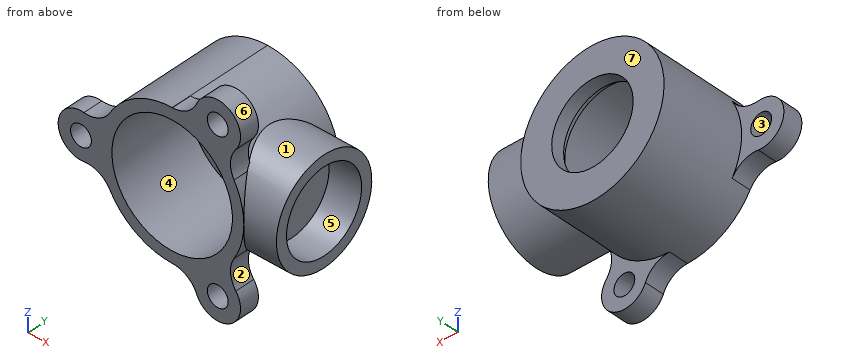
from build123d import *
from build123d.topology import SkipClean

# Parameters (mm, degrees)
SKETCH_1_R          = 11
EXTRUDE_1_DEPTH     = 16
CUT_EXTRUDE_1_REACH = 24.316
SKETCH_2_R          = 6.25
SKETCH_3_R          = 9.25
CUT_EXTRUDE_2_DEPTH = 13
EXTRUDE_2_REACH     = 35.257
SKETCH_4_R          = 8
SKETCH_5_R          = 6.3
CUT_EXTRUDE_3_DEPTH = 5
SKETCH_6_R          = 1.6
EXTRUDE_3_DEPTH     = 3
SKETCH_7_R          = 7
CUT_EXTRUDE_4_DEPTH = 1


with BuildPart() as part:
    # 草图1 → 凸台-拉伸1 (new body)
    with BuildSketch(Plane(origin=(0, 0, 0), x_dir=(1, 0, 0), z_dir=(0, 1, 0))):
        with Locations(Location((0, 0, 0), (0, 0, 270))):
            Circle(SKETCH_1_R)
    extrude(amount=EXTRUDE_1_DEPTH)

    # 草图2 → 切除-拉伸1 (cut, up to next)
    with BuildSketch(Plane(origin=(0, 16, 0), x_dir=(1, 0, 0), z_dir=(0, 1, 0)), mode=Mode.PRIVATE) as cut_extrude_1_sk1:
        with Locations(Location((0, 0, 0), (0, 0, 270))):
            Circle(SKETCH_2_R)
    cut_extrude_1_tool1 = extrude(cut_extrude_1_sk1.sketch, amount=-CUT_EXTRUDE_1_REACH, mode=Mode.PRIVATE) & part.part
    add(cut_extrude_1_tool1.solids().sort_by_distance((0, 16, 0))[0], mode=Mode.SUBTRACT)

    # 草图3 → 切除-拉伸2 (cut)
    with BuildSketch(Plane.XZ):
        with Locations(Location((0, 0, 0), (0, 0, 270))):
            Circle(SKETCH_3_R)
    extrude(amount=-CUT_EXTRUDE_2_DEPTH, mode=Mode.SUBTRACT)

    # 草图4 → 凸台-拉伸2 (add, up to next)
    with BuildSketch(Plane(origin=(16, 0, 0), x_dir=(0, 0, -1), z_dir=(1, 0, 0)), mode=Mode.PRIVATE) as extrude_2_sk1:
        with Locations((0, 8)):
            Circle(SKETCH_4_R)
    extrude_2_tool1 = extrude(extrude_2_sk1.sketch, amount=-EXTRUDE_2_REACH, mode=Mode.PRIVATE) - part.part
    add(extrude_2_tool1.solids().sort_by_distance((16, 8, 0))[0])

    # 草图5 → 切除-拉伸3 (cut)
    with SkipClean():  # the faces are left unmerged after this step: merging them gives an invalid solid
        with BuildSketch(Plane(origin=(16, 0, 0), x_dir=(0, 0, -1), z_dir=(1, 0, 0))):
            with Locations((0, 8)):
                Circle(SKETCH_5_R)
        extrude(amount=-CUT_EXTRUDE_3_DEPTH, mode=Mode.SUBTRACT)

    # 草图6 → 凸台-拉伸3 (add)
    # profile 1 of 3: a face of its own
    with SkipClean():  # the faces are left unmerged after this step: merging them gives an invalid solid
        with BuildSketch(Plane.XZ):
            with BuildLine():
                ThreePointArc((-11, 0), (-10.632091471, 2.821104562), (-9.55297619, 5.453498501))
                ThreePointArc((-9.55297619, 5.453498501), (-11.247511613, 3.854105973), (-13.545833333, 3.470408137))
                ThreePointArc((-13.545833333, 3.470408137), (-17.5, 0), (-13.545833333, -3.470408137))
                ThreePointArc((-13.545833333, -3.470408137), (-11.247511613, -3.854105973), (-9.55297619, -5.453498501))
                ThreePointArc((-9.55297619, -5.453498501), (-10.632091471, -2.821104562), (-11, 0))
            make_face()
            with Locations(Location((-14, 0, 0), (0, 0, 270))):
                Circle(SKETCH_6_R, mode=Mode.SUBTRACT)
        # profile 2 of 3: a face of its own
        with BuildSketch(Plane.XZ):
            with BuildLine():
                ThreePointArc((9.778378275, 9.995831713), (8.75, 15.155444566), (3.767455058, 13.466239851))
                ThreePointArc((3.767455058, 13.466239851), (2.286002125, 11.667683773), (0.053619854, 10.999869313))
                ThreePointArc((0.053619854, 10.999869313), (5.5, 9.526279442), (9.499356337, 5.546370812))
                ThreePointArc((9.499356337, 5.546370812), (8.961509488, 7.8135778), (9.778378275, 9.995831713))
            make_face()
            with Locations(Location((7, 12.124355653, 0), (0, 0, 270))):
                Circle(SKETCH_6_R, mode=Mode.SUBTRACT)
        # profile 3 of 3: a face of its own
        with BuildSketch(Plane.XZ):
            with BuildLine():
                ThreePointArc((3.767455058, -13.466239851), (8.75, -15.155444566), (9.778378275, -9.995831713))
                ThreePointArc((9.778378275, -9.995831713), (8.961509488, -7.8135778), (9.499356337, -5.546370812))
                ThreePointArc((9.499356337, -5.546370812), (5.5, -9.526279442), (0.053619854, -10.999869313))
                ThreePointArc((0.053619854, -10.999869313), (2.286002125, -11.667683773), (3.767455058, -13.466239851))
            make_face()
            with Locations(Location((7, -12.124355653, 0), (0, 0, 270))):
                Circle(SKETCH_6_R, mode=Mode.SUBTRACT)
        extrude(amount=-EXTRUDE_3_DEPTH)

    # 草图7 → 切除-拉伸4 (cut)
    with SkipClean():  # the faces are left unmerged after this step: merging them gives an invalid solid
        with BuildSketch(Plane.XZ.offset(-13)):
            with Locations(Location((0, 0, 0), (0, 0, 270))):
                Circle(SKETCH_7_R)
        extrude(amount=-CUT_EXTRUDE_4_DEPTH, mode=Mode.SUBTRACT)


solid = part.part
The listing builds one solid part. Answer for the finished solid, in the listing's coordinates (mm). Face numbers are marked on the shaded views. A direction names the side the tool comes from. Round coordinates to 2 decimals unless told otherwise and drop trailing zeros. Order: outer loops, then holes, each group sorted by start corner. A loop starts at its lowest first (then second) coordinate and runs counter-clockwise, first axis right, second up. Notation, with made-up numbers: (12.5, 72) -> (53.5, 72) arc R21 ccw to (53.5, 84) -> close; hole circle Ø3 at (33.5, -3). An arc over 180 degrees is marked (long way). One line per item, written item: value.
Item 1: Straight lines are drawn through the part: L1, parallel to X at y = 2, z = -0.5; L2, parallel to Z at x = 9.5, y = 14; L3, parallel to X at y = 14.5, z = 0. For each, find the intervals that lie inside material, in ascending order.
Taken from the geometry:
L1: x = -17.46 to -15.52, -12.48 to -9.24, 9.24 to 11
L2: z = -5.55 to 5.55
L3: x = -11 to -6.25, 6.25 to 16
Item 2: Find section A-A, the plane x = -14. Give the vertices of the cut face in (y, z), then the cut area to 3 significant figures.
Taken from the geometry:
outline: (0, -3.5) -> (3, -3.5) -> (3, -1.6) -> (0, -1.6) -> close; (0, 1.6) -> (3, 1.6) -> (3, 3.5) -> (0, 3.5) -> close
area: 11.4 mm2
Item 3: Find section C-C, the plane z = -5. Give the vertices of the cut face in (x, y) (3 decimals), then the cut area to 3 significant figures.
Taken from the geometry:
outline: (-9.855, 0) -> (-7.782, 0) -> (-7.782, 13) -> (-4.899, 13) -> (-4.899, 14) -> (-3.75, 14) -> (-3.75, 16) -> (-9.798, 16) -> (-9.798, 3) -> (-9.855, 3) -> close; (3.75, 14) -> (4.899, 14) -> (4.899, 13) -> (7.782, 13) -> (7.782, 0) -> (9.798, 0) -> (9.798, 1.755) -> (16, 1.755) -> (16, 4.167) -> (11, 4.167) -> (11, 11.833) -> (16, 11.833) -> (16, 14.245) -> (9.798, 14.245) -> (9.798, 16) -> (3.75, 16) -> close
area: 126 mm2
Item 4: Find section D-D, the plane z = 8.5. Give the vertices of the cut face in (x, y), then the cut area to 3 significant figures.
Taken from the geometry:
outline: (-6.98, 0) -> (-3.65, 0) -> (-3.65, 13) -> (3.65, 13) -> (3.65, 0) -> (9.06, 0) -> (9.06, 3) -> (6.98, 3) -> (6.98, 16) -> (-6.98, 16) -> close
area: 135 mm2
Item 5: Find section B-B, the plane y = 8. Give the vertices of the cut face in (x, z), then the cut area to 3 significant figures.
Taken from the geometry:
outline: (7.55, -8) -> (16, -8) -> (16, -6.3) -> (11, -6.3) -> (11, 6.3) -> (16, 6.3) -> (16, 8) -> (7.55, 8) arc R11 ccw (long way) to start; hole circle Ø18.5 at (0, 0)
area: 145 mm2
Item 6: For the marked faces 1, 2, 3 and 4, determine the directions among +Z, -Z, +X, -X, +Y, -Y from which every point of the face is accessible in a straight line to the end or side of a thin tool.
Taken from the geometry:
face 1: +X
face 2: +X, -Y
face 3: +Y, -Y
face 4: -Y
Item 7: Given P1, Ø8, axis at x = -13, y = 1.5, coming from the +Z side; P2, Ø14.5, axis at x = 0, z = 0, coming from the -Y side; P3, Ø4, axis at y = 11, z = 0, coming from the +X side, each flat-ended and moving along its own axis, determine where each tip first touches the part or whether it passes through.
Taken from the geometry:
P1: stops at z = 6.32
P2: stops at y = 13
P3: stops at x = 11
Item 8: For a pull along Y with two mould halves and no side action, classify the marked faces 5, 6 and 7 as released by +Y, released by -Y, zero draft, split by the parting line, or undercut.
Taken from the geometry:
face 5: undercut
face 6: zero draft
face 7: released by +Y
